Build history of the part. All positions in model axes, mm. Give positions to 0.01 mm unless a question says otherwise; leave off trailing zeros. Loops run counter-clockwise (first coordinate to the right, second up) from the corner with the lowest first, then second, coordinate; pieces in that order, holes last.
1) Flat gauge pin, fed straight in: P1, Ø10, axis at x = 1397.5, z = -4.5, coming from the +Y side. Where does the tip first touch, or does it go through?
2) Band-saw the part on C-C on z = 4. List the corners of the cut face in (x, y).
3) Band-saw the part on A-A on y = 3.5. List the corners of the cut face in (x, z).
4) Wall check: line 1 (Z direction, x = 1098, y = 7); line 2 (Z direction, x = 548.5, y = 19.5). Give the ranges that are in metal, low to high.
```python
from build123d import *

# Parameters (mm, degrees)
BOSS_EXTRUDE1_DEPTH = 2717.8


with BuildPart() as part:
    # Sketch1 → Boss-Extrude1 (new body)
    with BuildSketch(Plane(origin=(0, 0, 0), x_dir=(0, 0, -1), z_dir=(1, 0, 0))):
        with BuildLine():
            Line((-18, -17), (-18, 17))
            ThreePointArc((-18, 17), (-17.707106781, 17.707106781), (-17, 18))
            Line((-17, 18), (-14.5, 18))
            ThreePointArc((-14.5, 18), (-13.792893219, 17.707106781), (-13.5, 17))
            Line((-13.5, 17), (-13.5, 14.4))
            ThreePointArc((-13.5, 14.4), (-13.207106781, 13.692893219), (-12.5, 13.4))
            Line((-12.5, 13.4), (-12, 13.4))
            ThreePointArc((-12, 13.4), (-11.292893219, 13.692893219), (-11, 14.4))
            Line((-11, 14.4), (-11, 19.5))
            ThreePointArc((-11, 19.5), (-11.292893219, 20.207106781), (-12, 20.5))
            Line((-12, 20.5), (-19.5, 20.5))
            ThreePointArc((-19.5, 20.5), (-20.207106781, 20.207106781), (-20.5, 19.5))
            Line((-20.5, 19.5), (-20.5, -19.5))
            ThreePointArc((-20.5, -19.5), (-20.207106781, -20.207106781), (-19.5, -20.5))
            Line((-19.5, -20.5), (19.5, -20.5))
            ThreePointArc((19.5, -20.5), (20.207106781, -20.207106781), (20.5, -19.5))
            Line((20.5, -19.5), (20.5, 19.5))
            ThreePointArc((20.5, 19.5), (20.207106781, 20.207106781), (19.5, 20.5))
            Line((19.5, 20.5), (12, 20.5))
            ThreePointArc((12, 20.5), (11.292893219, 20.207106781), (11, 19.5))
            Line((11, 19.5), (11, 14.4))
            ThreePointArc((11, 14.4), (11.292893219, 13.692893219), (12, 13.4))
            Line((12, 13.4), (12.5, 13.4))
            ThreePointArc((12.5, 13.4), (13.207106781, 13.692893219), (13.5, 14.4))
            Line((13.5, 14.4), (13.5, 17))
            ThreePointArc((13.5, 17), (13.792893219, 17.707106781), (14.5, 18))
            Line((14.5, 18), (17, 18))
            ThreePointArc((17, 18), (17.707106781, 17.707106781), (18, 17))
            Line((18, 17), (18, -17))
            ThreePointArc((18, -17), (17.707106781, -17.707106781), (17, -18))
            Line((17, -18), (-17, -18))
            ThreePointArc((-17, -18), (-17.707106781, -17.707106781), (-18, -17))
        make_face()
    extrude(amount=BOSS_EXTRUDE1_DEPTH)


solid = part.part
```
Findings below:
1. P1: stops at y = -18
2. outline: (0, -20.5) - (2717.8, -20.5) - (2717.8, -18) - (0, -18) - close
3. outline: (0, -20.5) - (2717.8, -20.5) - (2717.8, -18) - (0, -18) - close; (0, 18) - (2717.8, 18) - (2717.8, 20.5) - (0, 20.5) - close
4. line 1: z = -20.5 to -18, 18 to 20.5
4. line 2: z = -20.5 to -11, 11 to 20.5
